Can you work these out from the model? Positions are in its coordinate system, mm. A direction names the side the tool comes from. Coordinates: 2 decimals unless noted, no trailing zeros. Loops run counter-clockwise (first coordinate to the right, second up) from the corner with the lowest first, then second, coordinate; pieces in that order, holes last. Notation, with made-up numbers: M 14,-21 L 29,-21 A16 cw 29,-17 Z; hole C 51.5,49 d11. An arc over 180 degrees is marked long. Answer as a JSON object with one key per item and string values. Group by question number.
Item 1: Suppose I cut it at D-D (x = 5.5). Write out the boundary of the cut face in (y, z).
Item 2: We'd pull the mould along X, two halves only. Please class faces 1 (the flat face through (0, -2.5, 5)), 2 (the cylindrical face through (0, 0, -2)), 3 (the flat face through (0.5, 0, -5)): +X half, -X half, draft (parallel to the pull), parting line (faces both ways), or undercut.
Item 3: I'm going to push flat-ended pins straight in: pin 1 Ø1.5 at (x, z) = (4, -1.5) entering from +Y; pin 2 Ø2.5 at (y, z) = (0.5, 5.5) entering from +X; pin 3 Ø1.4 at (x, y) = (-6, 0.5) entering from -Z; pin 4 Ø1.4 at (y, z) = (1, 4) entering from -X. Where does each tip first touch, or does it pass through?
Item 4: Suppose I cut it at B-B (y = 1.2). Write out the boundary of the cut face in (x, z), then the cut area to 3 significant figures.
Item 5: If I drill on line 1 (Z direction, x = 0, y = -0.4); line 2 (X direction, y = 1.3, z = -6.75), over which ranges is the centre line in solid material (lowest first)?
Item 6: Suppose I cut it at A-A (z = 0). Write out the boundary of the cut face in (x, y), then the cut area to 3 significant figures.
Item 7: Suppose I cut it at C-C (x = 0). Write out the boundary of the cut face in (y, z).
Item 8: Which directions (+Z, -Z, +X, -X, +Y, -Y) give clear straight access to the entire face, cutting with the end or side of a thin tool? Please do faces 4 (the cylindrical face through (0, 2, -3)), 5 (the flat face through (-5, -2.5, 0)), 6 (the flat face through (-0.5, 0, 5)), 7 (the flat face through (-0.5, 0, -5)), 8 (the cylindrical face through (0, -2, -3)).
```python
from build123d import *

# Parameters (mm, degrees)
F1_DEPTH = 2.5
F0_R     = 2
F2_DEPTH = 1


with BuildPart() as f1:
    # F0 (on Front) → F1 (new body, symmetric)
    with BuildSketch(Plane.XZ):
        with BuildLine():
            ThreePointArc((-0.5, 2.9580398915), (0, 3), (0.5, 2.9580398915))
            Line((0.5, 2.9580398915), (0.5, 7.7080398915))
            Line((0.5, 7.7080398915), (-0.5, 7.7080398915))
            Line((-0.5, 7.7080398915), (-0.5, 2.9580398915))
        make_face()
    extrude(amount=F1_DEPTH, both=True)



with BuildPart() as f1b:
    # F0 (on Front) → F1, piece 2 (new body, symmetric)
    with BuildSketch(Plane.XZ):
        with BuildLine():
            ThreePointArc((-2.9580398915, -0.5), (-3, 0), (-2.9580398915, 0.5))
            Line((-2.9580398915, 0.5), (-7.7080398915, 0.5))
            Line((-7.7080398915, 0.5), (-7.7080398915, -0.5))
            Line((-7.7080398915, -0.5), (-2.9580398915, -0.5))
        make_face()
    extrude(amount=F1_DEPTH, both=True)


with BuildPart() as f1c:
    # F0 (on Front) → F1, piece 3 (new body, symmetric)
    with BuildSketch(Plane.XZ):
        with BuildLine():
            Line((0.5, -7.7080398915), (0.5, -2.9580398915))
            ThreePointArc((0.5, -2.9580398915), (0, -3), (-0.5, -2.9580398915))
            Line((-0.5, -2.9580398915), (-0.5, -7.7080398915))
            Line((-0.5, -7.7080398915), (0.5, -7.7080398915))
        make_face()
    extrude(amount=F1_DEPTH, both=True)


with BuildPart() as f1d:
    # F0 (on Front) → F1, piece 4 (new body, symmetric)
    with BuildSketch(Plane.XZ):
        with BuildLine():
            ThreePointArc((2.9580398915, 0.5), (2.9894915684, 0.2508787808), (3, 0))
            ThreePointArc((3, 0), (2.9894915684, -0.2508787808), (2.9580398915, -0.5))
            Line((2.9580398915, -0.5), (7.7080398915, -0.5))
            Line((7.7080398915, -0.5), (7.7080398915, 0.5))
            Line((7.7080398915, 0.5), (2.9580398915, 0.5))
        make_face()
    extrude(amount=F1_DEPTH, both=True)


with BuildPart() as f1_1:
    add(f1.part)

    add(f1b.part)  # F2 merges F1b

    add(f1c.part)  # F2 merges F1c

    add(f1d.part)  # F2 merges F1d
    # F0 (on Front) → F2 (join, symmetric)
    with BuildSketch(Plane.XZ):
        with BuildLine():
            ThreePointArc((2.9580398915, -0.5), (2.9894915684, -0.2508787808), (3, 0))
            ThreePointArc((3, 0), (2.9894915684, 0.2508787808), (2.9580398915, 0.5))
            ThreePointArc((2.9580398915, 0.5), (2.1213203436, 2.1213203436), (0.5, 2.9580398915))
            ThreePointArc((0.5, 2.9580398915), (0, 3), (-0.5, 2.9580398915))
            ThreePointArc((-0.5, 2.9580398915), (-2.1213203436, 2.1213203436), (-2.9580398915, 0.5))
            ThreePointArc((-2.9580398915, 0.5), (-3, 0), (-2.9580398915, -0.5))
            ThreePointArc((-2.9580398915, -0.5), (-2.1213203436, -2.1213203436), (-0.5, -2.9580398915))
            ThreePointArc((-0.5, -2.9580398915), (0, -3), (0.5, -2.9580398915))
            ThreePointArc((0.5, -2.9580398915), (2.1213203436, -2.1213203436), (2.9580398915, -0.5))
        make_face()
        Circle(F0_R, mode=Mode.SUBTRACT)
    extrude(amount=F2_DEPTH, both=True)


solid = f1_1.part
```
From the geometry:
{
 "1": {"outline": "M -2.5,-0.5 L 2.5,-0.5 L 2.5,0.5 L -2.5,0.5 Z"},
 "2": {"face 1": "draft", "face 2": "undercut", "face 3": "+X half"},
 "3": {"pin 1": "through", "pin 2": "x = 0.5", "pin 3": "z = -0.5", "pin 4": "x = -0.5"},
 "4": {"outline": "M -7.71,-0.5 L -2.96,-0.5 A3 cw -2.96,0.5 L -7.71,0.5 Z; M -0.5,-7.71 L 0.5,-7.71 L 0.5,-2.96 A3 cw -0.5,-2.96 Z; M -0.5,2.96 A3 cw 0.5,2.96 L 0.5,7.71 L -0.5,7.71 Z; M 2.96,-0.5 L 7.71,-0.5 L 7.71,0.5 L 2.96,0.5 A3 cw Z", "area": "18.9 mm2"},
 "5": {"line 1": "-7.71 to -2, 2 to 7.71", "line 2": "-0.5 to 0.5"},
 "6": {"outline": "M -7.71,-2.5 L -3,-2.5 L -3,-1 L -2,-1 L -2,1 L -3,1 L -3,2.5 L -7.71,2.5 Z; M 2,-1 L 3,-1 L 3,-2.5 L 7.71,-2.5 L 7.71,2.5 L 3,2.5 L 3,1 L 2,1 Z", "area": "51.1 mm2"},
 "7": {"outline": "M -2.5,-7.71 L 2.5,-7.71 L 2.5,-3 L 1,-3 L 1,-2 L -1,-2 L -1,-3 L -2.5,-3 Z; M -2.5,3 L -1,3 L -1,2 L 1,2 L 1,3 L 2.5,3 L 2.5,7.71 L -2.5,7.71 Z"},
 "8": {"face 4": "+Y", "face 5": "+Z, -Z, +X, -X, -Y", "face 6": "+Z, -X, +Y, -Y", "face 7": "-Z, -X, +Y, -Y", "face 8": "-Y"}
}
